Geometry check sheet. Reference: the model listing, model coordinates, mm. A direction names the side the tool comes from. Give positions to 0.01 mm unless a question says otherwise; leave off trailing zeros. Order: outer loops, then holes, each group sorted by start corner. A loop starts at its lowest first (then second) coordinate and runs counter-clockwise, first axis right, second up.
Autodesk Fusion 360 part; units mm, degrees
sketch "Sketch1" plane through (0, 0, 0) normal (0, 0, 1) x (1, 0, 0)
  line L0 (36.0002, -9.75) -> (67.0101, -9.75)
  line L1 (67.0002, 9.75) -> (36.0002, 9.75)
  line L2 (67.0101, -4.75) -> (56.25, -4.75)
  arc A0 (56.25, 4.75) -> (51.5, 0) centre (56.25, 0) ccw
  line L3 (67.0101, -4.75) -> (67.0101, -9.75)
  line L4 (36.0002, 9.75) -> (36.0002, -9.75)
  arc A1 (51.5, 0) -> (56.25, -4.75) centre (56.25, 0) ccw
  line L5 (56.25, 4.75) -> (67.0002, 4.75)
  line L6 (67.0002, 4.75) -> (67.0002, 9.75)
  line L7 (0, 0) -> (36.0002, 0)
  point P0 (51.5001, 4.75)
  dimension "d7" = 4.75
  dimension "d8" = 4.75
  dimension "d9" = 4.75
  dimension "d10" = 31
  dimension "d11" = 19.5
extrude "Extrude1" add sketch "Sketch1" along normal blind 4
sketch "Sketch2" plane through (0, 0, 4) normal (0, 0, 1) x (-1, 0, 0)
  line L0 (-56.25, -4.75) -> (-67.0002, -4.75)
  line L1 (-67.0002, -4.75) -> (-67.0002, -9.75)
  line L2 (-67.0101, 9.75) -> (-67.0101, 4.75)
  line L3 (-67.0101, 4.75) -> (-56.25, 4.75)
  arc A0 (-51.5, 0) -> (-56.25, 4.75) centre (-56.25, 0) ccw
  arc A1 (-56.25, -4.75) -> (-51.5, 0) centre (-56.25, 0) ccw
  circle A2 centre (0, 0) radius 49.5
  circle A3 centre (0, 0) radius 19.05
  dimension "d14" = 99
  dimension "d15" = 38.1
extrude "Extrude2" add sketch "Sketch2" along normal blind 72
sketch "Sketch3" plane through (0, 0, 76) normal (0, 0, 1) x (-1, 0, 0)
  circle A0 centre (0, 0) radius 19.05
  circle A1 centre (0, 0) radius 49.5
  circle A2 centre (0, 0) radius 19.05
  circle A3 centre (0, 0) radius 26
extrude "Extrude3" add sketch "Sketch3" along normal blind 0.5 contours A3
sketch "Sketch4" plane through (0, 0, 4) normal (0, 0, -1) x (1, 0, 0)
  line L0 (36.0002, 9.75) -> (48.5303, 9.75)
  arc A0 (48.5303, 9.75) -> (48.5303, -9.75) centre (0, 0) ccw
  line L1 (48.5303, -9.75) -> (36.0002, -9.75)
  line L2 (36.0002, -9.75) -> (36.0002, 9.75)
  circle A1 centre (0, 0) radius 19.05
  line L3 (0, 0) -> (39.0512, 0) construction
  line L4 (29.6134, 29.6134) -> (23.9565, 35.2703)
  line L5 (29.6134, 29.6134) -> (35.2703, 23.9565)
  line L6 (23.9565, 35.2703) -> (26.785, 38.0987)
  line L7 (35.2703, 23.9565) -> (38.0987, 26.785)
  line L8 (38.0987, 26.785) -> (26.785, 38.0987)
  line L9 (-29.6134, 29.6134) -> (-35.2703, 23.9565)
  line L10 (-35.2703, 23.9565) -> (-38.0987, 26.785)
  line L11 (-26.785, 38.0987) -> (-38.0987, 26.785)
  line L12 (-23.9565, 35.2703) -> (-26.785, 38.0987)
  line L13 (-29.6134, 29.6134) -> (-23.9565, 35.2703)
  line L14 (-29.6134, -29.6134) -> (-23.9565, -35.2703)
  line L15 (-23.9565, -35.2703) -> (-26.785, -38.0987)
  line L16 (-38.0987, -26.785) -> (-26.785, -38.0987)
  line L17 (-35.2703, -23.9565) -> (-38.0987, -26.785)
  line L18 (-29.6134, -29.6134) -> (-35.2703, -23.9565)
  line L19 (29.6134, -29.6134) -> (35.2703, -23.9565)
  line L20 (35.2703, -23.9565) -> (38.0987, -26.785)
  line L21 (26.785, -38.0987) -> (38.0987, -26.785)
  line L22 (23.9565, -35.2703) -> (26.785, -38.0987)
  line L23 (29.6134, -29.6134) -> (23.9565, -35.2703)
  dimension "d24" = 8
  dimension "d25" = 8
  dimension "d28" = 360
extrude "Extrude4" add sketch "Sketch4" along normal blind 15 contours L4 L5 L6 L7 L8 | L9 L10 L11 L12 L13 | L14 L15 L16 L17 L18 | L19 L20 L21 L22 L23
sketch "Sketch5" plane through (0, 0, 76.5) normal (0, 0, 1) x (-1, 0, 0)
  circle A0 centre (0, 0) radius 19.05
  circle A1 centre (0, 0) radius 30
  circle A2 centre (0, 0) radius 19.05
  dimension "d31" = 60
extrude "Extrude5" add sketch "Sketch5" along normal blind 8
ref_plane "WorkPlane1" through (30, 0, 80.0207) normal (1, 0, 0) x (0, -1, 0)
sketch "Sketch6" plane through (30, 0, 0) normal (1, 0, 0) x (0, 1, 0)
  circle A0 centre (0, 80.5) radius 2
  dimension "d35" = 4
extrude "Extrude6" cut sketch "Sketch6" against normal blind 15.5
pattern_circular "C-Pattern1" count 4 over 360 about axis through (0, 0, 4) along (0, 0, 1) of "Extrude6"
equation "rotary_connect_length = 72 mm"
equation "d17 = rotary_connect_length"
equation "rotary_connect_space = 0.5 mm"
equation "rotary_connect_rotor_size = 8.5 mm"
equation "d21 = rotary_connect_space"
equation "d32 = rotary_connect_rotor_size - rotary_connect_space"
Item 1: Set-up check for faces 4 (the flat face through (29.534, 29.693, -3.395)), 5 (the flat face through (32.363, 32.521, -3.395)), 6 (the flat face through (-32.521, 32.363, -3.395)), 7 (the flat face through (25.351, -36.665, -3.395)): record each of +Z, -Z, +X, -X, +Y, -Y from which the full face is reachable in a straight line by a thin tool's end or side.
Reported:
face 4: -Z
face 5: -Z, +X, +Y
face 6: -Z, -X, +Y
face 7: -Z, -Y
Item 2: Sectioned sample at A-A (z = 2). Give the number of separate pieces and of enclosed holes in the cut face, and give its area (3 significant figures).
Reported:
separate pieces: 5
enclosed holes: 0
area: 723 mm2
Item 3: Scan lines: L1, parallel to Z at x = 27.75, y = 0; L2, parallel to X at y = 0, z = 31; L3, parallel to Z at x = -1.5, y = 27.5. Record each from-to range of solid material in increasing order.
Reported:
L1: z = 4 to 76, 76.5 to 78.5, 82.5 to 84.5
L2: x = -49.5 to -19.05, 19.05 to 49.5
L3: z = 4 to 76, 76.5 to 79.18, 81.82 to 84.5
Item 4: Sectioned sample at B-B (y = 0). Enter the section's corners in (x, z), and give its area (3 significant figures).
Reported:
outline: (-49.5, 4) - (-19.05, 4) - (-19.05, 78.5) - (-30, 78.5) - (-30, 76.5) - (-26, 76.5) - (-26, 76) - (-49.5, 76) - close; (-30, 82.5) - (-19.05, 82.5) - (-19.05, 84.5) - (-30, 84.5) - close; (19.05, 4) - (36, 4) - (36, 0) - (51.5, 0) - (51.5, 4) - (49.5, 4) - (49.5, 76) - (26, 76) - (26, 76.5) - (30, 76.5) - (30, 78.5) - (19.05, 78.5) - close; (19.05, 82.5) - (30, 82.5) - (30, 84.5) - (19.05, 84.5) - close
area: 4,540 mm2
Item 5: Gauge pin test, flat ends, axial feed: pin 1 (5 mm diameter, centred on x = 0, z = 80.5, fed in from +Y); pin 2 (1.5 mm diameter, centred on y = 6, z = 53, fed in from -X); pin 3 (2 mm diameter, centred on y = -6.5, z = 48.5, fed in from +X). Record the tip position at first contact, or that the pin passes through.
Reported:
pin 1: stops at y = 30
pin 2: stops at x = -49.22
pin 3: stops at x = 49.19
Item 6: Sectioned sample at C-C (x = 0). Enter the section's corners in (y, z).
Reported:
outline: (-49.5, 4) - (-19.05, 4) - (-19.05, 78.5) - (-30, 78.5) - (-30, 76.5) - (-26, 76.5) - (-26, 76) - (-49.5, 76) - close; (-30, 82.5) - (-19.05, 82.5) - (-19.05, 84.5) - (-30, 84.5) - close; (19.05, 4) - (49.5, 4) - (49.5, 76) - (26, 76) - (26, 76.5) - (30, 76.5) - (30, 78.5) - (19.05, 78.5) - close; (19.05, 82.5) - (30, 82.5) - (30, 84.5) - (19.05, 84.5) - close
Item 7: Sectioned sample at D-D (y = -22.5). Enter the section's corners in (x, z).
Reported:
outline: (-44.09, 4) - (44.09, 4) - (44.09, 76) - (13.03, 76) - (13.03, 76.5) - (19.84, 76.5) - (19.84, 84.5) - (-19.84, 84.5) - (-19.84, 76.5) - (-13.03, 76.5) - (-13.03, 76) - (-44.09, 76) - close; hole circle Ø4 at (0, 80.5)
Item 8: Draft check along Z on faces 1 (the flat face through (67, 7, 2)), 2 (the flat face through (48, 0, 0)), 3 (the cylindrical face through (-0.26, -24.55, 82.483)). Enter one of: released by +Z, released by -Z, zero draft, split by the parting line, or undercut.
Reported:
face 1: zero draft
face 2: released by -Z
face 3: undercut
